```python
from build123d import *

# Parameters (mm, degrees)
F0_R     = 38.158283
F1_DEPTH = 72.74499
F2_R     = 5.08
F3_R     = 14.290577
F4_DEPTH = 15.7517
F5_R     = 1.524


with BuildPart() as f1:
    # F0 (on Top) → F1 (new body)
    with BuildSketch(Plane.XY):
        Circle(F0_R)
    extrude(amount=F1_DEPTH)

    # F2
    f2_edges = [f1.edges().sort_by_distance(p)[0] for p in [
        (-38.158283, 0, 72.74499),
        (-38.158283, 0, 0),
    ]]
    fillet(f2_edges, radius=F2_R)

    # F3 (on face) → F4 (join)
    with BuildSketch(Plane.XY.offset(72.74499)):
        Circle(F3_R)
    extrude(amount=F4_DEPTH)

    # F5
    f5_edges = [f1.edges().sort_by_distance(p)[0] for p in [
        (-14.290577, 0, 88.49669),
    ]]
    fillet(f5_edges, radius=F5_R)


solid = f1.part
```
The model under review builds one solid part; all positions refer to its coordinate system, in mm. A direction names the side the tool comes from. Round coordinates to 2 decimals unless told otherwise and drop trailing zeros. Order: outer loops, then holes, each group sorted by start corner. A loop starts at its lowest first (then second) coordinate and runs counter-clockwise, first axis right, second up. Notation, with made-up numbers: (16, -12) -> (73, -12) arc R29 ccw to (73, 20) -> close; hole circle Ø1 at (-36.75, 46). An arc over 180 degrees is marked (long way). Use a Markdown table: item, result.
Q1. We need section A-A on x = 0. Write out the cut boundary in (y, z) (3 decimals).
Values:
| item | result |
|---|---|
| outline | (-38.158, 5.08) arc R5.08 ccw to (-33.078, 0) -> (33.078, 0) arc R5.08 ccw to (38.158, 5.08) -> (38.158, 67.665) arc R5.08 ccw to (33.078, 72.745) -> (14.291, 72.745) -> (14.291, 86.973) arc R1.524 ccw to (12.767, 88.497) -> (-12.767, 88.497) arc R1.524 ccw to (-14.291, 86.973) -> (-14.291, 72.745) -> (-33.078, 72.745) arc R5.08 ccw to (-38.158, 67.665) -> close |
Q2. We need section D-D on z = 70. Write out the cut boundary in (x, y), then the cut area to 3 significant figures.
Values:
| item | result |
|---|---|
| outline | circle Ø75.18 at (0, 0) |
| area | 4,440 mm^2 |
Q3. Clearance check with flat-ended pins moving along their axes: P1, Ø3, axis at y = -11, z = 65, coming from the +X side; P2, Ø3, axis at x = -27.5, z = 30.5, coming from the -Y side; P3, Ø8, axis at y = -4.5, z = 32.5, coming from the -X side (3 decimals); P4, Ø5, axis at y = 17.5, z = 77, coming from the -X side. State where each tip first meets the part, or that it passes through.
Values:
| item | result |
|---|---|
| P1 | stops at x = 36.96 |
| P2 | stops at y = -27.93 |
| P3 | stops at x = -38.155 |
| P4 | passes through |
Q4. We need section C-C on z = 44.5. Write out the cut boundary in (x, y).
Values:
| item | result |
|---|---|
| outline | circle Ø76.32 at (0, 0) |
Q5. Tool access review of faces 1 (the cylindrical face through (-3.1, -13.95, 79.76)), 2 (the flat face through (0, 0, 0)): name each direction out of +Z, -Z, +X, -X, +Y, -Y from which nothing blocks a thin tool from reaching the whole face with its end or side.
Values:
| item | result |
|---|---|
| face 1 | +Z |
| face 2 | -Z, +X, -X, +Y, -Y |
Q6. For line 1 (X direction, y = -0.5, z = 41.5) (3 decimals); line 2 (Z direction, x = -10.5, y = -13); line 3 (Z direction, x = -22, y = 26.5), list the stretches that pass through material, from the lowest coordinate up.
Values:
| item | result |
|---|---|
| line 1 | x = -38.155 to 38.155 |
| line 2 | z = 0 to 72.74 |
| line 3 | z = 0.19 to 72.56 |
